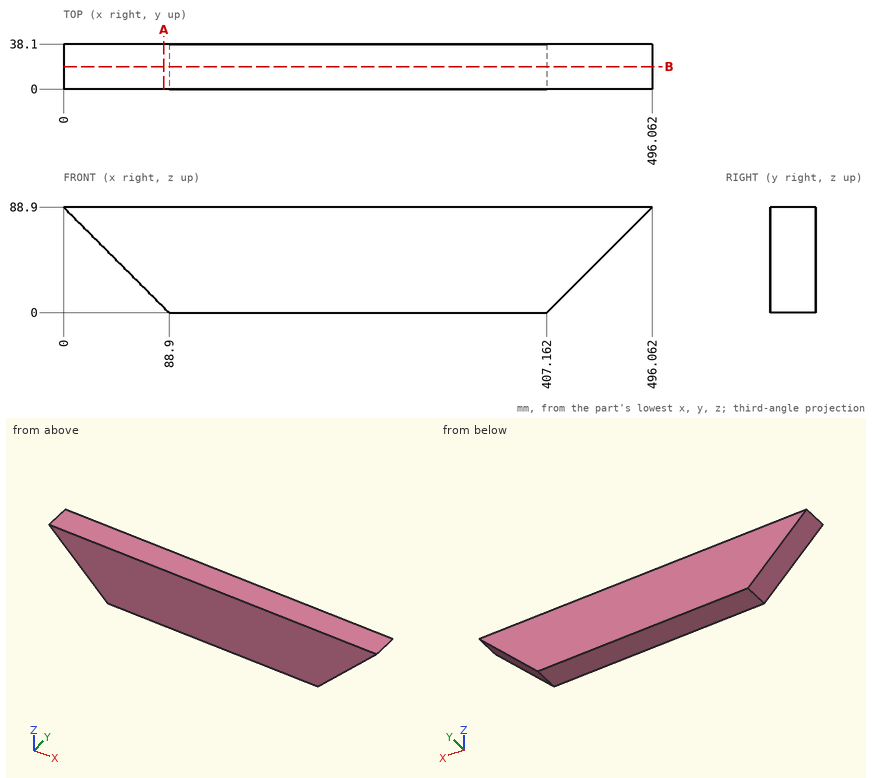
Drawing for the job (mm, zero at the part's lowest x, y, z). Round coordinates to 2 decimals unless told otherwise and drop trailing zeros. Write each loop counter-clockwise with the first axis right and the second up, starting at its lowest first coordinate (ties: lowest second). Pieces come first, ordered by that corner, then holes. Notation, with made-up numbers: M -13,-27 L 43,-27 A23 ccw 43,-17 Z; hole C -23,7 d7. An arc over 180 degrees is marked long. Answer in a Markdown table with one row per item.
1. Saw through at A-A (x = 84.5). List the corners of the cut face in (y, z).
Geometry check:
| item | result |
|---|---|
| outline | M 0,4.4 L 38.1,4.4 L 38.1,88.9 L 0,88.9 Z |
2. Flat gauge pins, fed straight in: P1, Ø4, axis at y = 24.5, z = 33, coming from the +X side; P2, Ø8, axis at y = 24.5, z = 54.5, coming from the +X side. Where does each tip first touch, or does it go through?
Geometry check:
| item | result |
|---|---|
| P1 | x = 442.16 |
| P2 | x = 465.66 |
3. Probe L1, parallel to X at y = 19, z = 11.5; L2, parallel to X at y = 8, z = 40; L3, parallel to Z at x = 65, y = 18. List the from-to ranges inside material, lowest first. Write a range as [from, to].
Geometry check:
| item | result |
|---|---|
| L1 | [77.4, 418.66] |
| L2 | [48.9, 447.16] |
| L3 | [23.9, 88.9] |
4. Saw through at B-B (y = 19). List the corners of the cut face in (x, z), and give its area (3 significant figures).
Geometry check:
| item | result |
|---|---|
| outline | M 0,88.9 L 88.9,0 L 407.16,0 L 496.06,88.9 Z |
| area | 36,200 mm2 |
